Check sheet for the modelled part. Datum: model origin and axes. Units: mm. A direction names the side the tool comes from. Round coordinates to 2 decimals unless told otherwise and drop trailing zeros. Write each loop counter-clockwise with the first axis right and the second up, starting at its lowest first coordinate (ties: lowest second). Pieces come first, ordered by that corner, then holes. Notation, with made-up numbers: (63, 16.5) -> (103, 16.5) arc R26 ccw to (103, 53.5) -> close; hole circle Ø3 at (28, 58.5). An arc over 180 degrees is marked (long way). Answer as a JSON object with one key per item and string values. Group by question number.
Autodesk Inventor part; units mm, degrees
ref_plane "YZ Plane" through (0, 0, 0) normal (1, 0, 0) x (0, 1, 0)
ref_plane "XZ Plane" through (0, 0, 0) normal (0, 1, 0) x (-1, 0, 0)
ref_plane "XY Plane" through (0, 0, 0) normal (0, 0, 1) x (1, 0, 0)
sketch "Sketch1" plane through (0, 0, 0) normal (0, 0, 1) x (1, 0, 0)
  circle A0 centre (0, 0) radius 50
  circle A1 centre (0, 0) radius 35
  dimension "d0" = 100
  dimension "d1" = 70
extrude "Extrusion1" add sketch "Sketch1" along normal blind 5.5
sketch "Sketch4" plane through (0, 0, 5.5) normal (0, 0, 1) x (1, 0, 0)
  line L0 (39.75, 2.75) -> (45.25, 2.75)
  line L1 (45.25, 2.75) -> (45.25, -2.75)
  line L2 (45.25, -2.75) -> (39.75, -2.75)
  line L3 (39.75, -2.75) -> (39.75, 2.75)
  line L4 (-39.75, -2.75) -> (-45.25, -2.75)
  line L5 (-45.25, -2.75) -> (-45.25, 2.75)
  line L6 (-45.25, 2.75) -> (-39.75, 2.75)
  line L7 (-39.75, 2.75) -> (-39.75, -2.75)
  point P0 (0, 0)
  dimension "d13" = 5.5
  dimension "d14" = 5.5
  dimension "d17" = 360
extrude "Extrusion3" cut sketch "Sketch4" against normal blind 10
sketch "Sketch5" plane through (0, 0, 5.5) normal (0, 0, 1) x (1, 0, 0)
  circle A0 centre (0, 0) radius 50
  line L0 (34.763, 35.938) -> (41.7155, 43.1255)
  line L1 (30.9949, 39.2341) -> (38.1218, 46.6018)
  line L2 (38.1218, 46.6018) -> (41.7155, 43.1255)
  line L3 (-34.763, 35.938) -> (-41.7155, 43.1255)
  line L4 (-30.9949, 39.2341) -> (-38.1218, 46.6018)
  line L5 (-38.1218, 46.6018) -> (-41.7155, 43.1255)
  arc A1 (-34.763, 35.938) -> (-30.9949, 39.2341) centre (-33.5607, 38.3654) ccw
  arc A2 (30.9949, 39.2341) -> (34.763, 35.938) centre (32.7963, 37.4916) ccw
  dimension "d21" = 10
  dimension "d22" = 5
extrude "Extrusion4" add sketch "Sketch5" against normal blind 5.5 contours A0 L1 L2 L0 | L3 L5 L4 A0 | A0 A1
properties part number "central"
(1) Section check A-A on x = 0. Record the cut outline in (y, z), then the cut area to 3 significant figures.
(2) Go/stop test with flat-tipped pins: pin 1 Ø1.6 at (x, z) = (-41, 3.5) entering from +Y; pin 2 Ø3 at (x, z) = (42, 3.5) entering from +Y. Record where each tip stops, or that it passes through.
(3) Release check for a two-part mould opening along X. For faces 4 (the cylindrical face through (-28, 21, 3)), 5 (the flat face through (38.19, 39.48, 2.79)), 6 (the flat face through (10, 34, 5.5)), 7 (the cylindrical face through (1.661, -49.972, 2.712)) record: pulls with the +X half, pulls with the -X half, needs draft (parallel to the pull), parting line crosses it, or undercut.
(4) Section check D-D on z = 3.05. Record the cut outline in (x, y).
(5) Section check B-B on y = 0. Record the cut outline in (x, z).
(6) Scan lines: line 1 along X through (y, z) = (-0.5, 3.25); line 2 along Y through (x, z) = (0, 2.35); line 3 along Y through (x, z) = (-30, 2). Record each from-to range of solid material in increasing order.
(7) Access from +Z, -Z, +X, -X, +Y, -Y to the whole of each face (thin tool, end or side, straight path). Record for faces 1 (the flat face through (-38.19, 39.48, 2.79)), 2 (the flat face through (45.25, 0, 3)), 3 (the flat face through (-34.51, 42.87, 2.79)).
(8) Section check C-C on y = 16. Record the cut outline in (x, z).
Data:
{
 "1": {"outline": "(-50, 0) -> (-35, 0) -> (-35, 5.5) -> (-50, 5.5) -> close; (35, 0) -> (50, 0) -> (50, 5.5) -> (35, 5.5) -> close", "area": "165 mm²"},
 "2": {"pin 1": "stops at y = 44.59", "pin 2": "stops at y = 44.3"},
 "3": {"face 4": "undercut", "face 5": "pulls with the +X half", "face 6": "needs draft", "face 7": "parting line crosses it"},
 "4": {"outline": "(-41.72, 43.13) -> (-34.76, 35.94) arc R50 ccw (long way) to (34.76, 35.94) -> (41.72, 43.13) -> (38.12, 46.6) -> (30.99, 39.23) arc R50 ccw to (-30.99, 39.23) -> (-38.12, 46.6) -> close; hole (-45.25, -2.75) -> (-39.75, -2.75) -> (-39.75, 2.75) -> (-45.25, 2.75) -> close; hole circle Ø70 at (0, 0); hole (39.75, -2.75) -> (45.25, -2.75) -> (45.25, 2.75) -> (39.75, 2.75) -> close"},
 "5": {"outline": "(-50, 0) -> (-45.25, 0) -> (-45.25, 5.5) -> (-50, 5.5) -> close; (-39.75, 0) -> (-35, 0) -> (-35, 5.5) -> (-39.75, 5.5) -> close; (35, 0) -> (39.75, 0) -> (39.75, 5.5) -> (35, 5.5) -> close; (45.25, 0) -> (50, 0) -> (50, 5.5) -> (45.25, 5.5) -> close"},
 "6": {"line 1": "x = -50 to -45.25, -39.75 to -35, 35 to 39.75, 45.25 to 50", "line 2": "y = -50 to -35, 35 to 50", "line 3": "y = -40 to -18.03, 18.03 to 40"},
 "7": {"face 1": "+Z, -Z, -X", "face 2": "+Z, -Z", "face 3": "+Z, -Z, +Y"},
 "8": {"outline": "(-47.37, 0) -> (-31.13, 0) -> (-31.13, 5.5) -> (-47.37, 5.5) -> close; (31.13, 0) -> (47.37, 0) -> (47.37, 5.5) -> (31.13, 5.5) -> close"}
}
